Source: CAD feature listing. Evaluate the final solid. Frame: model axes, mm. A direction names the side the tool comes from. Round coordinates to 2 decimals unless told otherwise and drop trailing zeros. Order: outer loops, then holes, each group sorted by start corner. A loop starts at its lowest first (then second) coordinate and runs counter-clockwise, first axis right, second up. Notation, with made-up numbers: (88, 88) -> (102, 88) arc R35 cw to (102, 123) -> close; hole circle Ø11 at (9, 65). An arc over 180 degrees is marked (long way). Use a Markdown table: item, result. Add a question column.
```python
from build123d import *

# Parameters (mm, degrees)
SKETCH1_R           = 2.4892
BOSS_EXTRUDE1_DEPTH = 2.5


with BuildPart() as part:
    # Sketch1 → Boss-Extrude1 (new body)
    with BuildSketch(Plane.XY):
        with BuildLine():
            Line((-1.6002, -57.15), (1.6002, -57.15))
            ThreePointArc((1.6002, -57.15), (3.84526403, -56.22006403), (4.7752, -53.975))
            Line((4.7752, -53.975), (4.7752, 1.6002))
            ThreePointArc((4.7752, 1.6002), (3.84526403, 3.84526403), (1.6002, 4.7752))
            Line((1.6002, 4.7752), (-53.975, 4.7752))
            ThreePointArc((-53.975, 4.7752), (-56.22006403, 3.84526403), (-57.15, 1.6002))
            Line((-57.15, 1.6002), (-57.15, -9.525))
            ThreePointArc((-57.15, -9.525), (-56.22006403, -11.77006403), (-53.975, -12.7))
            Line((-53.975, -12.7), (-7.9502, -12.7))
            ThreePointArc((-7.9502, -12.7), (-5.70513597, -13.62993597), (-4.7752, -15.875))
            Line((-4.7752, -15.875), (-4.7752, -53.975))
            ThreePointArc((-4.7752, -53.975), (-3.84526403, -56.22006403), (-1.6002, -57.15))
        make_face()
        with Locations((-12.7, 0)):
            Circle(SKETCH1_R, mode=Mode.SUBTRACT)
        Circle(SKETCH1_R, mode=Mode.SUBTRACT)
        with Locations((-25.4, 0)):
            Circle(SKETCH1_R, mode=Mode.SUBTRACT)
        with Locations((-38.1, 0)):
            Circle(SKETCH1_R, mode=Mode.SUBTRACT)
        with Locations((-50.8, 0)):
            Circle(SKETCH1_R, mode=Mode.SUBTRACT)
        with Locations((0, -12.7)):
            Circle(SKETCH1_R, mode=Mode.SUBTRACT)
        with Locations((0, -25.4)):
            Circle(SKETCH1_R, mode=Mode.SUBTRACT)
        with Locations((0, -38.1)):
            Circle(SKETCH1_R, mode=Mode.SUBTRACT)
        with Locations((0, -50.8)):
            Circle(SKETCH1_R, mode=Mode.SUBTRACT)
    extrude(amount=-BOSS_EXTRUDE1_DEPTH)


solid = part.part
```
1) Section D-D on x = -12.7. Output: boundary loops of the cut face in (y, z).
2) Section B-B on y = -50.8. Output: boundary loops of the cut face in (x, z).
3) Reachability of faces 1 (the flat face through (-26, 4.775, -1)), 2 (the flat face through (-31, -12.7, -1)) from +Z, -Z, +X, -X, +Y, -Y: full face, straight path, thin tool, end or side. Return the list, or none.
4) Line query: probe 1 along Y at (x, z) = (0, -1.3); probe 2 along Y at (x, z) = (-1, -1.7); probe 3 along Y at (x, z) = (-19, -2.2). Output: solid intervals per line, ascending. Write a range as from..to.
5) Section C-C on x = 0.5. Output: boundary loops of the cut face in (y, z), then the cut area to 3 significant figures.
6) Section A-A on y = 0. Output: boundary loops of the cut face in (x, z).
7) First-contact query: pin 1 Ø8 at (x, y) = (-38.1, 0) entering from +Z; pin 2 Ø1 at (x, z) = (-11.5, -1) entering from -Y. Flat tips, straight axial feed; report the tip coordinate or a pass-through.
Conclusion:
| question | item | result |
|---|---|---|
| 1 | outline | (-12.7, -2.5) -> (-2.49, -2.5) -> (-2.49, 0) -> (-12.7, 0) -> close; (2.49, -2.5) -> (4.78, -2.5) -> (4.78, 0) -> (2.49, 0) -> close |
| 2 | outline | (-4.78, -2.5) -> (-2.49, -2.5) -> (-2.49, 0) -> (-4.78, 0) -> close; (2.49, -2.5) -> (4.78, -2.5) -> (4.78, 0) -> (2.49, 0) -> close |
| 3 | face 1 | +Z, -Z, +X, -X, +Y |
| 3 | face 2 | +Z, -Z, -X, -Y |
| 4 | probe 1 | y = -57.15..-53.29, -48.31..-40.59, -35.61..-27.89, -22.91..-15.19, -10.21..-2.49, 2.49..4.78 |
| 4 | probe 2 | y = -57.15..-53.08, -48.52..-40.38, -35.82..-27.68, -23.12..-14.98, -10.42..-2.28, 2.28..4.78 |
| 4 | probe 3 | y = -12.7..4.78 |
| 5 | outline | (-57.15, -2.5) -> (-53.24, -2.5) -> (-53.24, 0) -> (-57.15, 0) -> close; (-48.36, -2.5) -> (-40.54, -2.5) -> (-40.54, 0) -> (-48.36, 0) -> close; (-35.66, -2.5) -> (-27.84, -2.5) -> (-27.84, 0) -> (-35.66, 0) -> close; (-22.96, -2.5) -> (-15.14, -2.5) -> (-15.14, 0) -> (-22.96, 0) -> close; (-10.26, -2.5) -> (-2.44, -2.5) -> (-2.44, 0) -> (-10.26, 0) -> close; (2.44, -2.5) -> (4.78, -2.5) -> (4.78, 0) -> (2.44, 0) -> close |
| 5 | area | 93.9 mm^2 |
| 6 | outline | (-57.15, -2.5) -> (-53.29, -2.5) -> (-53.29, 0) -> (-57.15, 0) -> close; (-48.31, -2.5) -> (-40.59, -2.5) -> (-40.59, 0) -> (-48.31, 0) -> close; (-35.61, -2.5) -> (-27.89, -2.5) -> (-27.89, 0) -> (-35.61, 0) -> close; (-22.91, -2.5) -> (-15.19, -2.5) -> (-15.19, 0) -> (-22.91, 0) -> close; (-10.21, -2.5) -> (-2.49, -2.5) -> (-2.49, 0) -> (-10.21, 0) -> close; (2.49, -2.5) -> (4.78, -2.5) -> (4.78, 0) -> (2.49, 0) -> close |
| 7 | pin 1 | stops at z = 0 |
| 7 | pin 2 | stops at y = -12.7 |
